Geometry check sheet. Reference: the model listing, model coordinates, mm. Give positions to 0.01 mm unless a question says otherwise; leave off trailing zeros. Order: outer loops, then holes, each group sorted by start corner. A loop starts at its lowest first (then second) coordinate and runs counter-clockwise, first axis right, second up. Notation, with made-up numbers: M 41,-16.5 L 45,-16.5 A31 ccw 45,15.5 Z; hole C -5,19.5 d7. An arc over 180 degrees is marked long. Answer as CSV lines item,"result".
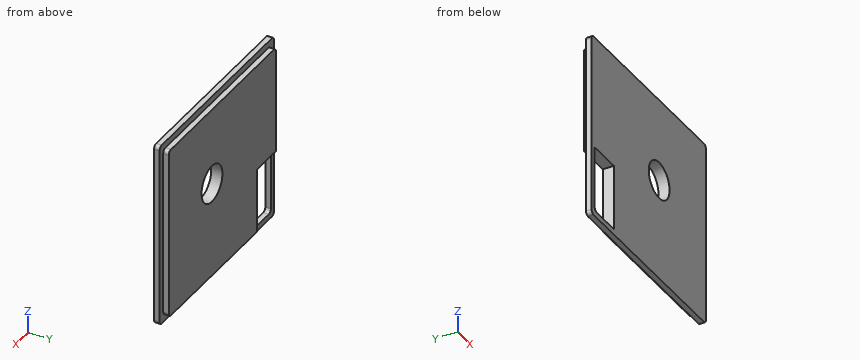
Autodesk Inventor part; units mm, degrees
ref_plane "YZ Plane" through (0, 0, 0) normal (1, 0, 0) x (0, 1, 0)
ref_plane "XZ Plane" through (0, 0, 0) normal (0, 1, 0) x (-1, 0, 0)
ref_plane "XY Plane" through (0, 0, 0) normal (0, 0, 1) x (1, 0, 0)
sketch "Sketch1" plane through (0, 0, 0) normal (0, 1, 0) x (-1, 0, 0)
  line L0 (0, 0) -> (110, 0)
  line L1 (110, 0) -> (110, -100)
  line L2 (110, -100) -> (0, -100)
  line L3 (0, -100) -> (0, 0)
  dimension "d0" = 100
  dimension "d1" = 110
extrude "Extrusion1" add sketch "Sketch1" along normal blind 3
sketch "Sketch2" plane through (0, 3, 0) normal (0, 1, 0) x (1, 0, 0)
  line L0 (-106.5, 3.5) -> (-3.5, 3.5)
  line L1 (-3.5, 3.5) -> (-3.5, 96.5)
  line L2 (-3.5, 96.5) -> (-106.5, 96.5)
  line L3 (-106.5, 96.5) -> (-106.5, 3.5)
  line L4 (-110, 100) -> (-110, 0)
  line L5 (-110, 0) -> (0, 0)
  line L6 (0, 100) -> (-110, 100)
  line L7 (0, 0) -> (0, 100)
  dimension "d4" = 3.5
  dimension "d5" = 3.5
  dimension "d6" = 3.5
  dimension "d7" = 3.5
extrude "Extrusion2" add sketch "Sketch2" along normal blind 3 contours L3 L2 L1 L0
fillet "Fillet1" radius 2 8 edges at (0, 1.5, 0) (-3.5, 4.5, -3.5) (-110, 1.5, 0) (-106.5, 4.5, -3.5) (-106.5, 4.5, -96.5) (-110, 1.5, -100) (-3.5, 4.5, -96.5) (0, 1.5, -100)
sketch "Sketch3" plane through (0, 0, 0) normal (0, -1, 0) x (1, 0, 0)
  line L0 (-107, -97) -> (-88.5, -97)
  line L1 (-88.5, -97) -> (-88.5, -61.5)
  line L2 (-88.5, -61.5) -> (-107, -61.5)
  line L3 (-107, -61.5) -> (-107, -97)
  line L4 (-108, -100) -> (-2, -100)
  line L5 (-110, -2) -> (-110, -98)
  point P0 (0, 0)
  dimension "d11" = 35.5
  dimension "d12" = 18.5
  dimension "d13" = 3
  dimension "d14" = 3
extrude "Extrusion3" cut sketch "Sketch3" against normal blind 10
fillet "Fillet2" radius 2 1 edges at (-107, 1.5, -97)
sketch "Sketch4" plane through (0, 0, 0) normal (0, -1, 0) x (1, 0, 0)
  circle A0 centre (-45, -45) radius 10
  line L0 (0, -98) -> (0, -2)
  line L1 (-2, 0) -> (-108, 0)
  point P0 (0, 0)
  dimension "d18" = 20
  dimension "d20" = 45
  dimension "d21" = 45
extrude "Extrusion4" cut sketch "Sketch4" against normal blind 10
sketch "Sketch5" plane through (0, 0, 0) normal (0, -1, 0) x (1, 0, 0)
  point P0 (0, 0)
properties part number "StaniceBoxTop"
(1) Section check D-D on x = -84.5. Enter the section's corners in (y, z).
The answers:
outline,"M 0,-100 L 3,-100 L 3,-96.5 L 6,-96.5 L 6,-3.5 L 3,-3.5 L 3,0 L 0,0 Z"
(2) Section check B-B on x = -45. Enter the section's corners in (y, z), then the cut area to 3 significant figures.
The answers:
outline,"M 0,-100 L 3,-100 L 3,-96.5 L 6,-96.5 L 6,-55 L 0,-55 Z; M 0,-35 L 6,-35 L 6,-3.5 L 3,-3.5 L 3,0 L 0,0 Z"
area,"459 mm2"
(3) Material ranges on line 1 (Z direction, x = -45, y = 1.55); line 2 (Z direction, x = -99.5, y = 0.9); line 3 (X direction, y = 5.65, z = -25), recorded low to high.
The answers:
line 1,"z = -100 to -55, -35 to 0"
line 2,"z = -100 to -97, -61.5 to 0"
line 3,"x = -106.5 to -3.5"
(4) Section check C-C on z = -45. Enter the section's corners in (x, y), then the cut area to 3 significant figures.
The answers:
outline,"M -110,0 L -55,0 L -55,6 L -106.5,6 L -106.5,3 L -110,3 Z; M -35,0 L 0,0 L 0,3 L -3.5,3 L -3.5,6 L -35,6 Z"
area,"519 mm2"
(5) Section check A-A on y = 1.1. Enter the section's corners in (x, z).
The answers:
outline,"M -110,-98 A2 ccw -108,-100 L -2,-100 A2 ccw 0,-98 L 0,-2 A2 ccw -2,0 L -108,0 A2 ccw -110,-2 Z; hole M -107,-95 A2 ccw -105,-97 L -88.5,-97 L -88.5,-61.5 L -107,-61.5 Z; hole C -45,-45 d20"
(6) Gauge pin test, flat ends, axial feed: P1, Ø1.5, axis at x = -65.5, y = 4, coming from the +Z side; P2, Ø1.5, axis at y = 5, z = -54, coming from the +X side. Record the tip position at first contact, or that the pin passes through.
The answers:
P1,"stops at z = -3.5"
P2,"stops at x = -3.5"
